The listing builds one solid part. Answer for the finished solid, in the listing's coordinates (mm). A direction names the side the tool comes from. Round coordinates to 2 decimals unless told otherwise and drop trailing zeros. Loops run counter-clockwise (first coordinate to the right, second up) from the corner with the lowest first, then second, coordinate; pieces in that order, holes last. Notation, with made-up numbers: (53, 57) -> (98, 57) arc R17 ccw to (98, 63) -> close; hole circle Ø8 at (-24, 34). An arc over 180 degrees is marked (long way). One line per question, with ' | ' between items.
from build123d import *

# Parameters (mm, degrees)
F0_R     = 50
F1_DEPTH = 10
F2_T     = -2.5
F3_R     = 25
F4_DEPTH = 25


with BuildPart() as f1:
    # F0 (on Top) → F1 (new body)
    with BuildSketch(Plane.XY):
        Circle(F0_R)
    extrude(amount=F1_DEPTH)

    # F2
    f2_openings = [f1.faces().sort_by_distance(p)[0] for p in [
        (0, 0, 0),
    ]]
    offset(amount=F2_T, openings=f2_openings)

    # F3 (on face) → F4 (cut)
    with BuildSketch(Plane.XY.offset(10)):
        Circle(F3_R)
    extrude(amount=-F4_DEPTH, mode=Mode.SUBTRACT)


solid = f1.part
Q1. For faces 4 (the face through (23.846, 7.509, 8.768)), 5 (the face through (-10.3, -46.37, 3.7)), determine the directions among +Z, -Z, +X, -X, +Y, -Y from which every point of the face is accessible in a straight line to the end or side of a thin tool.
Numbers:
face 4: +Z, -Z | face 5: -Z
Q2. A cutting plane is placed at A-A on y = 0. Give the vertices of the cut face in (x, z).
Numbers:
outline: (-50, 0) -> (-47.5, 0) -> (-47.5, 7.5) -> (-25, 7.5) -> (-25, 10) -> (-50, 10) -> close; (25, 7.5) -> (47.5, 7.5) -> (47.5, 0) -> (50, 0) -> (50, 10) -> (25, 10) -> close
Q3. A cutting plane is placed at D-D on y = -29.5. Give the vertices of the cut face in (x, z).
Numbers:
outline: (-40.37, 0) -> (-37.23, 0) -> (-37.23, 7.5) -> (37.23, 7.5) -> (37.23, 0) -> (40.37, 0) -> (40.37, 10) -> (-40.37, 10) -> close
Q4. A cutting plane is placed at C-C on z = 2.5. Give the vertices of the cut face in (x, y), plus the area to 3 significant figures.
Numbers:
outline: circle Ø100 at (0, 0); hole circle Ø95 at (0, 0) | area: 766 mm^2
Q5. For a pull along Y with two mould halves and no side action, classify faces 1 (the face through (47.69, 15.02, 4.93)), 2 (the face through (20, -20, 7.5)), 3 (the face through (44.2, -18.3, 0)) as pulls with the +Y half, pulls with the -Y half, needs draft (parallel to the pull), parting line crosses it, or undercut.
Numbers:
face 1: parting line crosses it | face 2: undercut | face 3: needs draft
Q6. Given pin 1 Ø6 at (y, z) = (11.5, 9) entering from -X; pin 2 Ø12 at (x, y) = (-4.5, 27) entering from -Z; pin 3 Ø6 at (y, z) = (-21, 4.5) entering from +X; pin 4 Ø8 at (x, y) = (18.5, -6.5) entering from +Z, each flat-ended and moving along its own axis, determine where each tip first touches the part or whether it passes through.
Numbers:
pin 1: x = -49.27 | pin 2: z = 7.5 | pin 3: x = 46.65 | pin 4: through
Q7. Find the intervals of material crossed by line 1 (Y direction, x = 0, z = 8.8); line 2 (Y direction, x = 0, z = 2.75); line 3 (Z direction, x = 12.5, y = -27), in increasing order. Write a range as from..to.
Numbers:
line 1: -50..-25, 25..50 | line 2: -50..-47.5, 47.5..50 | line 3: 7.5..10
